from build123d import *

# Parameters (mm, degrees)
SKETCH2_R           = 5
SKETCH2_R_2         = 4
BOSS_EXTRUDE1_DEPTH = 3
SKETCH7_R           = 100
CUT_EXTRUDE2_DEPTH  = 10


with BuildPart() as part:
    # Sketch2 → Boss-Extrude1 (new body)
    with BuildSketch(Plane.XY):
        with BuildLine():
            Line((-125, 140), (125, 140))
            ThreePointArc((125, 140), (135.606601718, 135.606601718), (140, 125))
            Line((140, 125), (140, -125))
            ThreePointArc((140, -125), (135.606601718, -135.606601718), (125, -140))
            Line((125, -140), (-125, -140))
            ThreePointArc((-125, -140), (-135.606601718, -135.606601718), (-140, -125))
            Line((-140, -125), (-140, 125))
            ThreePointArc((-140, 125), (-135.606601718, 135.606601718), (-125, 140))
        make_face()
        with Locations((-125, 125)):
            Circle(SKETCH2_R, mode=Mode.SUBTRACT)
        with Locations((0, 125)):
            Circle(SKETCH2_R, mode=Mode.SUBTRACT)
        with Locations((125, 125)):
            Circle(SKETCH2_R, mode=Mode.SUBTRACT)
        Circle(SKETCH2_R_2, mode=Mode.SUBTRACT)
        with Locations((125, 0)):
            Circle(SKETCH2_R, mode=Mode.SUBTRACT)
        with Locations((-125, 0)):
            Circle(SKETCH2_R, mode=Mode.SUBTRACT)
        with Locations((-125, -125)):
            Circle(SKETCH2_R, mode=Mode.SUBTRACT)
        with Locations((0, -125)):
            Circle(SKETCH2_R, mode=Mode.SUBTRACT)
        with Locations((125, -125)):
            Circle(SKETCH2_R, mode=Mode.SUBTRACT)
    extrude(amount=BOSS_EXTRUDE1_DEPTH)

    # Sketch7 → Cut-Extrude2 (cut)
    with BuildSketch(Plane.XY.offset(3)):
        Circle(SKETCH7_R)
    extrude(amount=-CUT_EXTRUDE2_DEPTH, mode=Mode.SUBTRACT)


solid = part.part
Check sheet for the modelled part. Datum: model origin and axes. Units: mm. Coordinates: 2 decimals unless noted, no trailing zeros. Write each loop counter-clockwise with the first axis right and the second up, starting at its lowest first coordinate (ties: lowest second). Pieces come first, ordered by that corner, then holes.
Item 1: Scan lines: probe 1 along Y at (x, z) = (-125, 2.3); probe 2 along Y at (x, z) = (0, 1.8); probe 3 along X at (y, z) = (-53, 2.5). Record each from-to range of solid material in increasing order.
Numbers:
probe 1: y = -140 to -130, -120 to -5, 5 to 120, 130 to 140
probe 2: y = -140 to -130, -120 to -100, 100 to 120, 130 to 140
probe 3: x = -140 to -84.8, 84.8 to 140
Item 2: Cross-section at A-A on y = 0. Record the boundary of the cut face in (x, z).
Numbers:
outline: (-140, 0) - (-130, 0) - (-130, 3) - (-140, 3) - close; (-120, 0) - (-100, 0) - (-100, 3) - (-120, 3) - close; (100, 0) - (120, 0) - (120, 3) - (100, 3) - close; (130, 0) - (140, 0) - (140, 3) - (130, 3) - close
Item 3: Cross-section at D-D on z = 0.9. Count the separate pieces of the cut face and the enclosed holes in it, then the cut area to 3 significant figures.
Numbers:
separate pieces: 1
enclosed holes: 9
area: 46,200 mm2
Item 4: Mould release check, pull along Y, two halves, no side actions. Record for faces 1 (the face through (129.77, 126.5, 1.48)), 2 (the face through (135.72, -135.49, 1.48)), 3 (the face through (-135.72, 135.49, 1.48)): released by +Y, released by -Y, zero draft, split by the parting line, or undercut.
Numbers:
face 1: undercut
face 2: released by -Y
face 3: released by +Y
Item 5: Cross-section at C-C on x = -69. Record the boundary of the cut face in (y, z), then the cut area to 3 significant figures.
Numbers:
outline: (-140, 0) - (-72.38, 0) - (-72.38, 3) - (-140, 3) - close; (72.38, 0) - (140, 0) - (140, 3) - (72.38, 3) - close
area: 406 mm2
